```python
from build123d import *

# Parameters (mm, degrees)
SKETCH_1_W      = 110
SKETCH_1_H      = 160
EXTRUDE_1_DEPTH = 3
EXTRUDE_2_DEPTH = 50
FILLET_1_R      = 5
CHAMFER_1_SIZE  = 4
FILLET_2_R      = 5
FILLET_3_R      = 5
FILLET_4_R      = 5.5


with BuildPart() as part:
    # 草图1 → 凸台-拉伸1 (new body)
    with BuildSketch(Plane(origin=(0, 0, 0), x_dir=(1, 0, 0), z_dir=(0, 1, 0))):
        with Locations((55, 80)):
            Rectangle(SKETCH_1_W, SKETCH_1_H)
    extrude(amount=EXTRUDE_1_DEPTH)

    # 草图2 → 凸台-拉伸2 (add)
    with BuildSketch(Plane(origin=(0, 3, 0), x_dir=(1, 0, 0), z_dir=(0, 1, 0))):
        Polygon((0, 0), (110, 0), (110, 3), (110, 160), (107, 160), (107, 3), (0, 3), align=None)
    extrude(amount=EXTRUDE_2_DEPTH)

    # 圆角1
    fillet_1_edges = [part.edges().sort_by_distance(p)[0] for p in [
        (107, 3, -81.5),
        (53.5, 3, -3),
    ]]
    fillet(fillet_1_edges, radius=FILLET_1_R)

    # 倒角1
    chamfer_1_edges = [part.edges().sort_by_distance(p)[0] for p in [
        (110, 0, -80),
        (55, 0, 0),
    ]]
    chamfer(chamfer_1_edges, length=CHAMFER_1_SIZE)

    # 圆角2
    fillet_2_edges = [part.edges().sort_by_distance(p)[0] for p in [
        (0, 1.5, -160),
    ]]
    fillet(fillet_2_edges, radius=FILLET_2_R)

    # 圆角3
    # the kernel refuses this fillet: 5 mm, written as the material it adds along each edge
    with BuildSketch(Plane(origin=(102, 8, -8), x_dir=(0, 0, 1), z_dir=(1, 0, 0))) as fillet_3_piece_1_section:
        Polygon((0, 0), (FILLET_3_R, 0), (FILLET_3_R, FILLET_3_R), (0, FILLET_3_R), align=None)
    fillet_3_piece_1 = extrude(amount=FILLET_3_R, mode=Mode.PRIVATE)
    fillet_3_piece_1 = fillet_3_piece_1 - Plane(origin=(102, 8, -8), x_dir=(0, 0.7071067811865475, -0.7071067811865475), z_dir=(1, 0, 0)) * Sphere(FILLET_3_R, mode=Mode.PRIVATE)
    add(fillet_3_piece_1)
    with BuildSketch(Plane(origin=(107, 8, -3), x_dir=(0, 0, -1), z_dir=(0, 1, 0))) as fillet_3_piece_2:
        with BuildLine():
            CenterArc((FILLET_3_R, FILLET_3_R), FILLET_3_R, 180, 90)
            Line((0, FILLET_3_R), (0, 0))
            Line((0, 0), (FILLET_3_R, 0))
        make_face()
    extrude(amount=45)

    # 圆角4
    fillet_4_edges = [part.edges().sort_by_distance(p)[0] for p in [
        (110, 28.5, 0),
    ]]
    fillet(fillet_4_edges, radius=FILLET_4_R)


solid = part.part
```
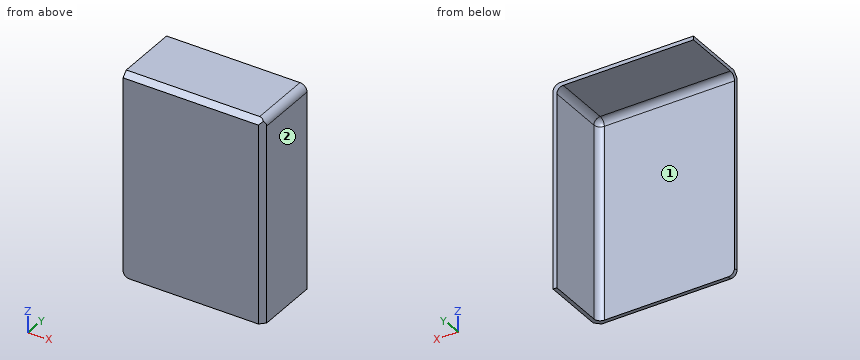
Geometry check sheet. Reference: the model listing, model coordinates, mm. Face numbers are marked on the shaded views. A direction names the side the tool comes from. Coordinates: 2 decimals unless noted, no trailing zeros. Write each loop counter-clockwise with the first axis right and the second up, starting at its lowest first coordinate (ties: lowest second). Pieces come first, ordered by that corner, then holes. Notation, with made-up numbers: M 19,-2 L 52,-2 A15 cw 52,25 Z; hole C 24,35.5 d10. An arc over 180 degrees is marked long. Answer as a JSON object with one key per item and string values.
1. Section check A-A, the plane z = -146. Enter the section's corners in (x, y).
Answers below:
{"outline": "M 0,0 L 106,0 L 110,4 L 110,53 L 107,53 L 107,8 A5 cw 102,3 L 0,3 Z"}
2. Scan lines: L1, parallel to X at y = 41.5, z = -16; L2, parallel to Y at x = 41, z = -20.5; L3, parallel to Z at x = 98, y = 40. Record each from-to range of solid material in increasing order.
Answers below:
{"L1": "x = 107 to 110", "L2": "y = 0 to 3", "L3": "z = -3 to 0"}
3. Section check B-B, the plane x = 34. Enter the section's corners in (y, z), plus the area to 3 significant figures.
Answers below:
{"outline": "M 0,-160 L 3,-160 L 3,-8 A5 cw 8,-3 L 53,-3 L 53,0 L 4,0 L 0,-4 Z", "area": "627 mm²"}
4. Tool access check on the marked faces 1 and 2. Record the directions out of +Z, -Z, +X, -X, +Y, -Y that give a thin tool (end or side, any length) a straight path to the whole face; none if there is none.
Answers below:
{"face 1": "-Z, -X, +Y", "face 2": "+Z, -Z, +X, +Y, -Y"}
5. Go/stop test with flat-tipped pins: pin 1 Ø12 at (y, z) = (24, -85) entering from -X; pin 2 Ø3 at (x, z) = (45, -60) entering from +Y; pin 3 Ø13.5 at (x, y) = (35.5, 36) entering from -Z. Record where each tip stops, or that it passes through.
Answers below:
{"pin 1": "stops at x = 107", "pin 2": "stops at y = 3", "pin 3": "stops at z = -3"}
